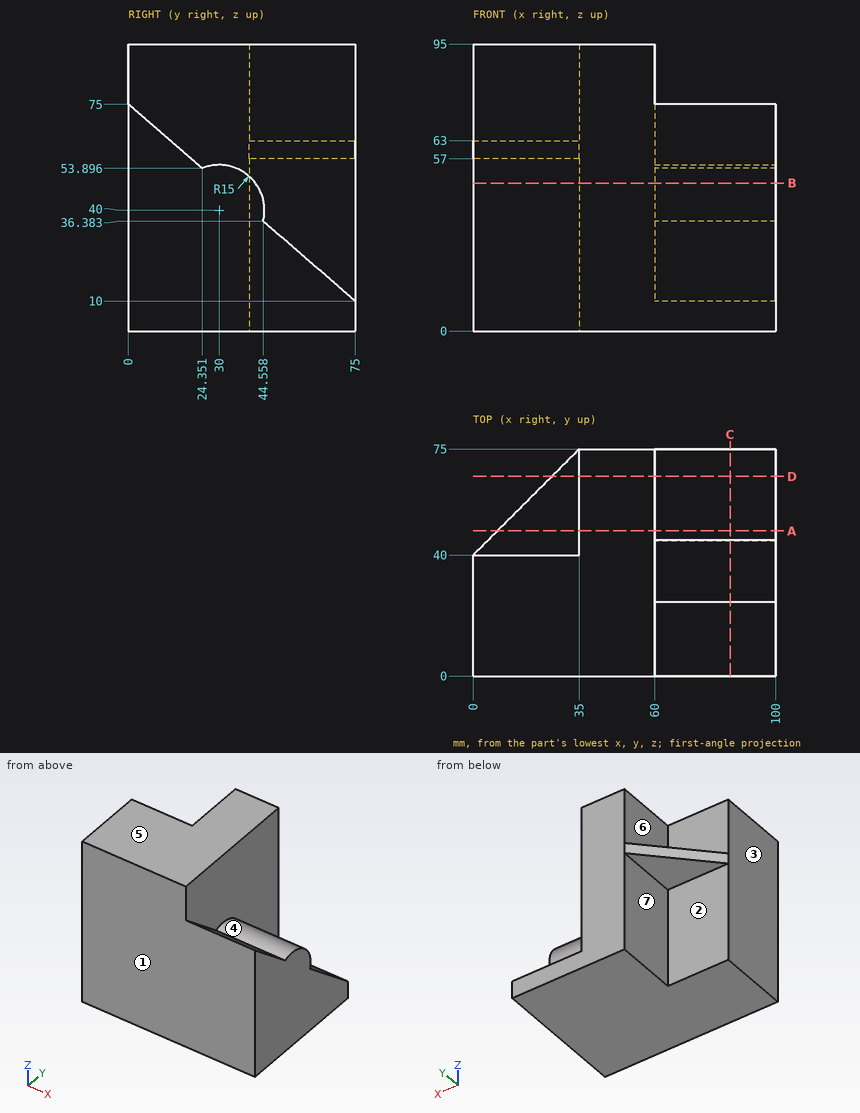
The figure shows three views and two pictorial views of one solid part (mm, origin at its lowest corner). Answer the questions. A direction names the side the tool comes from. Give positions to 0.01 mm unless a question says otherwise; leave off trailing zeros. Write each loop counter-clockwise with the first axis right and the second up, starting at its lowest first coordinate (ties: lowest second). Pieces come first, ordered by that corner, then holes. Notation, with made-up numbers: M 36,-36.75 L 43,-36.75 A21 cw 43,-12.75 Z; hole C -26,45 d11. An arc over 180 degrees is marked long. One line per item, written item: value. Start each with the question number.
(1) Determine the mould class of the marked faces 1, 2, 3 and 4 for opening direction Y: pulls with the +Y half, pulls with the -Y half, needs draft (parallel to the pull), parting line crosses it, or undercut.
(2) Find section D-D (y = 66). Determine the outline of the cut face in (x, z).
(3) Find the intervals of material crossed by line 1 (Y direction, x = 4, z = 80); line 2 (X direction, y = 55.5, z = 88); line 3 (Z direction, x = 25.5, y = 53), in increasing order.
(4) A tool of negligible diameter and unlimited length cuts with its end or side. For the marked faces 5, 6 and 7, from which of +Z, -Z, +X, -X, +Y, -Y can it reach the whole face along a straight path? Write none if from no direction.
(5) Flat-ended cylindrical pins translate along their axes: pin 1 Ø17.5 at (x, y) = (14.5, 59) entering from +Z; pin 2 Ø8 at (x, z) = (30, 44) entering from +Y; pin 3 Ø17.5 at (y, z) = (64.5, 41) entering from -X. Find the tip coordinate at first contact, or state that the pin passes through.
(6) Find section C-C (x = 85). Determine the outline of the cut face in (y, z) (1 decimal).
(7) Find section A-A (y = 48). Determine the outline of the cut face in (x, z), plus the area to 3 significant figures.
(8) Find section B-B (z = 49). Determine the outline of the cut face in (x, y), plus the area to 4 significant figures.
Results below:
1. face 1: pulls with the -Y half
1. face 2: pulls with the +Y half
1. face 3: needs draft
1. face 4: undercut
2. outline: M 26,57 L 35,57 L 35,0 L 100,0 L 100,17.8 L 60,17.8 L 60,95 L 35,95 L 35,63 L 26,63 Z
3. line 1: y = 0 to 40
3. line 2: x = 35 to 60
3. line 3: z = 57 to 63
4. face 5: +Z, +X, -X, +Y, -Y
4. face 6: +Z, -X, +Y
4. face 7: -Z, -X, +Y
5. pin 1: stops at z = 63
5. pin 2: stops at y = 40
5. pin 3: stops at x = 35
6. outline: M 0,0 L 75,0 L 75,10 L 44.6,36.4 A15 ccw 24.4,53.9 L 0,75 Z
7. outline: M 8,57 L 35,57 L 35,0 L 100,0 L 100,33.4 L 60,33.4 L 60,95 L 35,95 L 35,63 L 8,63 Z
7. area: 3,870 mm^2
8. outline: M 0,0 L 100,0 L 100,42 L 60,42 L 60,75 L 35,75 L 35,40 L 0,40 Z
8. area: 4,955 mm^2
